Design review of the part built by this model. Coordinates are the model's own, in mm. A direction names the side the tool comes from. Give positions to 0.01 mm unless a question says otherwise; leave off trailing zeros. Loops run counter-clockwise (first coordinate to the right, second up) from the corner with the lowest first, then second, coordinate; pieces in that order, holes last. Notation, with made-up numbers: (37.25, 89) -> (43.25, 89) arc R21 ccw to (43.25, 99) -> close; hole circle Ø1 at (1.25, 6). An arc over 180 degrees is marked (long way). Use a Markdown table: item, result. Add a question column.
1. Add section B-B (x = 6.95). State the section outline as (y, z) points, and give its area (3 significant figures).
2. To check wall thickness, follow line 1 (Y direction, x = 37, z = 2.1); line 2 (X direction, y = 5, z = 1.8); line 3 (Y direction, x = 28, z = 1.45). State the ranges of each line that lie inside material, in increasing order.
3. Add section C-C (y = 21.5). State the section outline as (x, z) points.
4. Add section A-A (x = 36.95). State the section outline as (y, z) points, and give its area (3 significant figures).
5. For pin 1 Ø1 at (y, z) = (21, 1) entering from -X; pin 2 Ø2 at (x, z) = (1, 2) entering from +Y; pin 3 Ø2 at (y, z) = (15, 1.5) entering from +X; pin 4 Ø2 at (y, z) = (1.5, 2.5) entering from +X, all flat-tipped, find the tip position at first contact; note any pin that passes through.
6. For faces 4 (the cylindrical face through (6.62, 30.18, 1.97)), 5 (the flat face through (8, 10, 2)), 6 (the flat face through (30.9, 9, 2)), 7 (the cylindrical face through (31.634, 31.713, 2.028)), list the 3-axis set-ups (+Z, -Z, +X, -X, +Y, -Y) from which the entire face can be reached by the end or side of a thin tool; tool diameter is ignored.
7. Add section D-D (z = 2.3). State the section outline as (x, y) points.
8. Draft analysis for pull direction Y (two halves, no side actions). For faces 1 (the flat face through (6, 7.5, 2)), 2 (the cylindrical face through (42.05, 31.4, 1.97)), 3 (the flat face through (0, 2, 2)), state which applies: pulls with the +Y half, pulls with the -Y half, needs draft (parallel to the pull), parting line crosses it, or undercut.
```python
from build123d import *

# Parameters (mm, degrees)
SKETCH2_R           = 1.5
BOSS_EXTRUDE1_DEPTH = 4
FILLET1_R           = 5


with BuildPart() as part:
    # Sketch2 → Boss-Extrude1 (new body)
    with BuildSketch(Plane.XY):
        with BuildLine():
            Line((0, 4), (0, 0))
            Line((0, 0), (38.9, 0))
            Line((38.9, 0), (38.9, 4))
            Line((38.9, 4), (34.9, 4))
            Line((34.9, 4), (34.9, 7.5))
            Line((34.9, 7.5), (30.9, 7.5))
            Line((30.9, 7.5), (30.9, 11.5))
            Line((30.9, 11.5), (41.95, 11.5))
            Line((41.95, 11.5), (41.95, 21.5))
            ThreePointArc((41.95, 21.5), (41.95, 31.5), (31.95, 31.5))
            Line((31.95, 31.5), (16.95, 31.5))
            ThreePointArc((16.95, 31.5), (-3.05, 31.5), (-3.05, 11.5))
            Line((-3.05, 11.5), (8, 11.5))
            Line((8, 11.5), (8, 7.5))
            Line((8, 7.5), (4, 7.5))
            Line((4, 7.5), (4, 4))
            Line((4, 4), (0, 4))
        make_face()
        with Locations((12.021067812, 30.283347099)):
            Circle(SKETCH2_R, mode=Mode.SUBTRACT)
        with Locations((6.95, 31.642135624)):
            Circle(SKETCH2_R, mode=Mode.SUBTRACT)
        with Locations((1.878932188, 30.283347099)):
            Circle(SKETCH2_R, mode=Mode.SUBTRACT)
        with Locations((-1.833347099, 26.571067812)):
            Circle(SKETCH2_R, mode=Mode.SUBTRACT)
        with Locations((15.733347099, 26.571067812)):
            Circle(SKETCH2_R, mode=Mode.SUBTRACT)
        with Locations((6.95, 21.5)):
            Circle(SKETCH2_R, mode=Mode.SUBTRACT)
        with Locations((36.95, 26.5)):
            Circle(SKETCH2_R, mode=Mode.SUBTRACT)
    extrude(amount=BOSS_EXTRUDE1_DEPTH)

    # Fillet1
    fillet1_edges = [part.edges().sort_by_distance(p)[0] for p in [
        (16.95, 31.5, 2),
        (31.95, 31.5, 2),
        (41.95, 21.5, 2),
    ]]
    fillet(fillet1_edges, radius=FILLET1_R)


solid = part.part
```
Taken from the geometry:
| question | item | result |
|---|---|---|
| 1 | outline | (0, 0) -> (7.5, 0) -> (7.5, 4) -> (0, 4) -> close; (11.5, 0) -> (20, 0) -> (20, 4) -> (11.5, 4) -> close; (23, 0) -> (30.14, 0) -> (30.14, 4) -> (23, 4) -> close; (33.14, 0) -> (35.64, 0) -> (35.64, 4) -> (33.14, 4) -> close |
| 1 | area | 103 mm^2 |
| 2 | line 1 | y = 0 to 4, 11.5 to 25, 28 to 33.57 |
| 2 | line 2 | x = 4 to 34.9 |
| 2 | line 3 | y = 0 to 31.5 |
| 3 | outline | (-7.19, 0) -> (5.45, 0) -> (5.45, 4) -> (-7.19, 4) -> close; (8.45, 0) -> (42.27, 0) -> (42.27, 4) -> (8.45, 4) -> close |
| 4 | outline | (0, 0) -> (4, 0) -> (4, 4) -> (0, 4) -> close; (11.5, 0) -> (25, 0) -> (25, 4) -> (11.5, 4) -> close; (28, 0) -> (33.57, 0) -> (33.57, 4) -> (28, 4) -> close |
| 4 | area | 92.3 mm^2 |
| 5 | pin 1 | stops at x = -7.19 |
| 5 | pin 2 | stops at y = 34.75 |
| 5 | pin 3 | stops at x = 41.95 |
| 5 | pin 4 | stops at x = 38.9 |
| 6 | face 4 | +Z, -Z |
| 6 | face 5 | +Z, -Z, -X |
| 6 | face 6 | +Z, -Z, +X |
| 6 | face 7 | +Z, -Z, +Y |
| 7 | outline | (-3.05, 11.5) -> (8, 11.5) -> (8, 7.5) -> (4, 7.5) -> (4, 4) -> (0, 4) -> (0, 0) -> (38.9, 0) -> (38.9, 4) -> (34.9, 4) -> (34.9, 7.5) -> (30.9, 7.5) -> (30.9, 11.5) -> (41.95, 11.5) -> (41.95, 19.74) arc R5 cw to (42.81, 22.54) arc R7.07 ccw to (32.99, 32.36) arc R5 cw to (30.19, 31.5) -> (18.84, 31.5) arc R5 cw to (15.74, 32.58) arc R14.14 ccw to start; hole circle Ø3 at (-1.83, 26.57); hole circle Ø3 at (1.88, 30.28); hole circle Ø3 at (6.95, 21.5); hole circle Ø3 at (6.95, 31.64); hole circle Ø3 at (12.02, 30.28); hole circle Ø3 at (15.73, 26.57); hole circle Ø3 at (36.95, 26.5) |
| 8 | face 1 | undercut |
| 8 | face 2 | parting line crosses it |
| 8 | face 3 | needs draft |
